Work out the finished part from the listing and answer in its coordinate system (mm). A direction names the side the tool comes from. Round coordinates to 2 decimals unless told otherwise and drop trailing zeros. Order: outer loops, then holes, each group sorted by start corner. A loop starts at its lowest first (then second) coordinate and runs counter-clockwise, first axis right, second up. Notation, with made-up numbers: (-39, -39) - (-25, -39) arc R27 cw to (-25, -12) - close; hole circle Ø7 at (-27, 76). An arc over 180 degrees is marked (long way). Put each result on its own line as item: value.
```python
from build123d import *

# Parameters (mm, degrees)
SKETCH3_R           = 4.2
CUT_EXTRUDE1_DEPTH  = 10
SKETCH6_W           = 13.7
SKETCH6_H           = 7
CUT_EXTRUDE8_DEPTH  = 59
CUT_EXTRUDE9_DEPTH  = 7
SKETCH8_W           = 2
SKETCH8_H           = 4
CUT_EXTRUDE10_DEPTH = 61


with BuildPart() as part:
    # Sketch2 → Revolve1 (revolve)
    with BuildSketch(Plane.XY, mode=Mode.PRIVATE) as revolve1_sk:
        Polygon((0, 20), (10, 20), (30, 0), (0, 0), align=None)
    revolve(revolve1_sk.sketch.rotate(Axis((0, 0, 0), (0, 1, 0)), 90), axis=Axis((0, 0, 0), (0, 1, 0)))

    # Sketch3 → Cut-Extrude1 (cut)
    with BuildSketch(Plane(origin=(0, 20, 0), x_dir=(1, 0, 0), z_dir=(0, 1, 0))):
        with Locations(Location((0, 0, 0), (0, 0, 270))):
            Circle(SKETCH3_R)
    extrude(amount=-CUT_EXTRUDE1_DEPTH, mode=Mode.SUBTRACT)

    # Sketch6 → Cut-Extrude8 (cut)
    with BuildSketch(Plane.XY):
        with Locations((0, 9.5)):
            Rectangle(SKETCH6_W, SKETCH6_H)
    extrude(amount=-CUT_EXTRUDE8_DEPTH, mode=Mode.SUBTRACT)

    # Sketch7 → Cut-Extrude9 (cut)
    with BuildSketch(Plane(origin=(0, 6, 0), x_dir=(1, 0, 0), z_dir=(0, 1, 0))):
        Polygon((6.85, -3.954849344), (6.85, 3.954849344), (0, 7.909698688), (-6.85, 3.954849344), (-6.85, -3.954849344), (0, -7.909698688), align=None)
    extrude(amount=CUT_EXTRUDE9_DEPTH, mode=Mode.SUBTRACT)

    # Sketch8 → Cut-Extrude10 (cut)
    with BuildSketch(Plane.XY):
        Rectangle(SKETCH8_W, SKETCH8_H)
    extrude(amount=-CUT_EXTRUDE10_DEPTH, mode=Mode.SUBTRACT)


solid = part.part
```
1) A cutting plane is placed at B-B on y = 6.75. Write down the section's boundary in (x, z), then the cut area to 3 significant figures.
Findings below:
outline: (-6.85, -22.22) - (-6.85, 3.95) - (0, 7.91) - (6.85, 3.95) - (6.85, -22.22) arc R23.25 ccw (long way) to start
area: 1,300 mm2
2) Given pin 1 Ø6 at (y, z) = (2.5, -17.5) entering from +X; pin 2 Ø1 at (y, z) = (1, -17) entering from +X; pin 3 Ø5.5 at (y, z) = (8, -7) entering from +X, each flat-ended and moving along its own axis, determine where each tip first touches the part or whether it passes through.
Findings below:
pin 1: stops at x = 25.48
pin 2: stops at x = 24.2
pin 3: stops at x = 23.84
3) For a pull along Y with two mould halves and no side action, classify faces 1 (the flat face through (-3.473, 9.451, 5.905)), 2 (the flat face through (0, 2, -14)), 3 (the flat face through (-1, 1, -15)), 4 (the flat face through (-6.85, 9, -6)) as pulls with the +Y half, pulls with the -Y half, needs draft (parallel to the pull), parting line crosses it, or undercut.
Findings below:
face 1: undercut
face 2: pulls with the -Y half
face 3: needs draft
face 4: undercut
4) A cutting plane is placed at A-A on y = 18.25. Write down the section's boundary in (x, z), then the cut area to 3 significant figures.
Findings below:
outline: circle Ø23.5 at (0, 0); hole circle Ø8.4 at (0, 0)
area: 378 mm2
5) Straight lines are drawn through the part: L1, parallel to X at y = 14.5, z = 0; L2, parallel to X at y = 18, z = 0; L3, parallel to Y at x = 4, z = -16. For each, find the intervals that lie inside material, in ascending order. Write a range as from..to.
Findings below:
L1: x = -15.5..-4.2, 4.2..15.5
L2: x = -12..-4.2, 4.2..12
L3: y = 0..6, 13..13.51
6) For faces 5 (the flat face through (0, 6, -8)), 6 (the cylindrical face through (1.262, 16.549, 4.006)), 7 (the flat face through (1, 1, -15)), determine the directions among +Z, -Z, +X, -X, +Y, -Y from which every point of the face is accessible in a straight line to the end or side of a thin tool.
Findings below:
face 5: -Z
face 6: +Y
face 7: -Z, -Y
